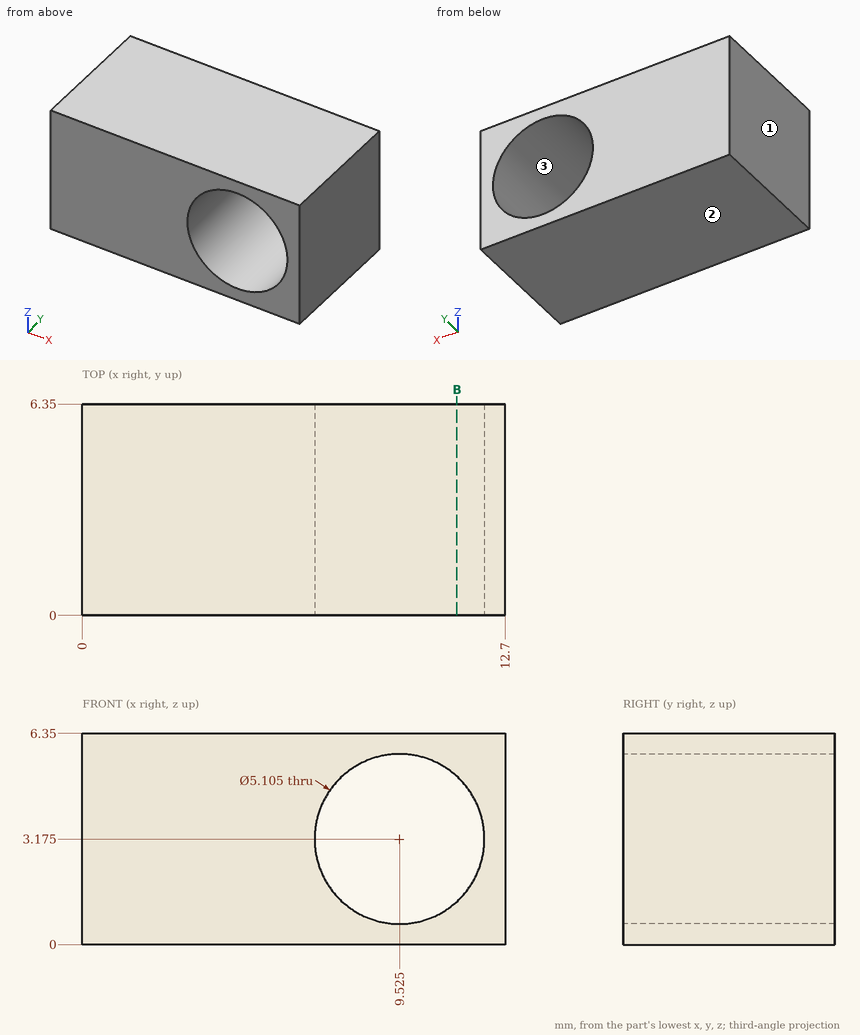
Design review of the part shown in the three views and the two pictorial views. Dimensions are in mm from the part's minimum x, y and z. Give positions to 0.01 mm unless a question says otherwise; leave off trailing zeros. Loops run counter-clockwise (first coordinate to the right, second up) from the corner with the lowest first, then second, coordinate; pieces in that order, holes last. Notation, with made-up numbers: (-19, 20) - (25, 20) arc R18 cw to (25, 48) - close; hole circle Ø2 at (-14.75, 5). An arc over 180 degrees is marked (long way). Answer as a JSON object with one key per item and string values.
Q1. Insertion check: pin 1 (1 mm diameter, centred on x = 11.5, z = 4, fed in from -Y). The pin has a flat end and moves straight along its axis. Give the tip position at first contact, or say it passes through.
Worked out:
{"pin 1": "stops at y = 0"}
Q2. Add section B-B on x = 11.25. State the section outline as (y, z) points.
Worked out:
{"outline": "(0, 0) - (6.35, 0) - (6.35, 1.29) - (0, 1.29) - close; (0, 5.06) - (6.35, 5.06) - (6.35, 6.35) - (0, 6.35) - close"}
Q3. Mouldability with a two-part tool opening along Z and no side actions: class the marked faces 1, 2 and 3 as +Z half, -Z half, draft (parallel to the pull), parting line (faces both ways), or undercut.
Worked out:
{"face 1": "draft", "face 2": "-Z half", "face 3": "undercut"}
Q4. To check wall thickness, follow line 1 along Z through (x, y) = (11, 2); line 2 along X through (y, z) = (4.5, 3.25); line 3 along X through (y, z) = (5.5, 3.75). State the ranges of each line that lie inside material, in increasing order.
Worked out:
{"line 1": "z = 0 to 1.09, 5.26 to 6.35", "line 2": "x = 0 to 6.97, 12.08 to 12.7", "line 3": "x = 0 to 7.04, 12.01 to 12.7"}
